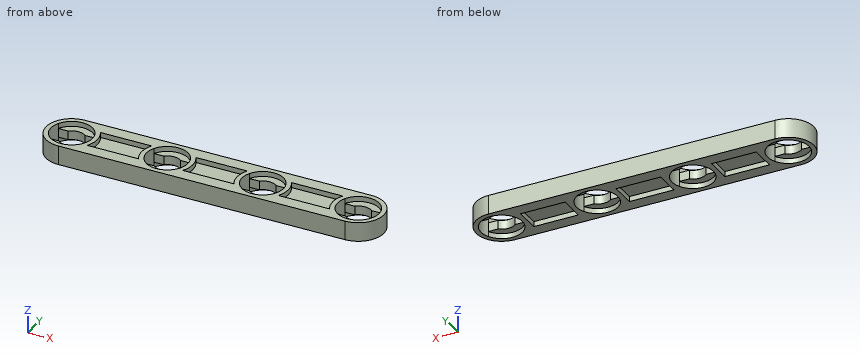
```python
from build123d import *

# Parameters (mm, degrees)
EXTRUDE_1_DEPTH          = 3
CUT_EXTRUDE_1_REACH      = 51.254
SKETCH_3_R               = 3.25
CUT_EXTRUDE_2_DEPTH      = 0.8
CUT_EXTRUDE_START        = -2.2
SKETCH_3_2_R             = 3.25
CUT_EXTRUDE_3_DEPTH      = 0.8
CUT_EXTRUDE_4_DEPTH      = 0.8
SKETCH_5_W               = 7
SKETCH_5_H               = 4
CUT_EXTRUDE_6_DEPTH      = 0.8
MIRROR_2_COPY_1_REACH    = 51.254
MIRROR_2_COPY_2_SKETCH_R = 3.25
MIRROR_2_COPY_2_DEPTH    = 0.8
MIRROR_START             = -2.2
MIRROR_2_COPY_3_SKETCH_R = 3.25
MIRROR_2_COPY_3_DEPTH    = 0.8


with BuildPart() as part:
    # 草图1 → 凸台-拉伸1 (new body)
    with BuildSketch(Plane.XY):
        with BuildLine():
            Line((0, 4), (45, 4))
            ThreePointArc((45, 4), (49, 0), (45, -4))
            Line((45, -4), (0, -4))
            ThreePointArc((0, -4), (-4, 0), (0, 4))
        make_face()
    extrude(amount=-EXTRUDE_1_DEPTH)

    # 草图2 → 切除-拉伸1 (cut, up to next)
    with BuildSketch(Plane.XY, mode=Mode.PRIVATE) as cut_extrude_1_sk1:
        with BuildLine():
            Line((1.322875656, -1.5), (2.883140649, -1.5))
            ThreePointArc((2.883140649, -1.5), (3.25, 0), (2.883140649, 1.5))
            Line((2.883140649, 1.5), (1.322875656, 1.5))
            ThreePointArc((1.322875656, 1.5), (0, 2), (-1.322875656, 1.5))
            Line((-1.322875656, 1.5), (-2.883140649, 1.5))
            ThreePointArc((-2.883140649, 1.5), (-3.25, 0), (-2.883140649, -1.5))
            Line((-2.883140649, -1.5), (-1.322875656, -1.5))
            ThreePointArc((-1.322875656, -1.5), (0, -2), (1.322875656, -1.5))
        make_face()
    cut_extrude_1_tool1 = extrude(cut_extrude_1_sk1.sketch, amount=-CUT_EXTRUDE_1_REACH, mode=Mode.PRIVATE) & part.part
    cut_extrude_1 = cut_extrude_1_tool1.solids().sort_by_distance((0, 0, 0))[0]
    add(cut_extrude_1, mode=Mode.SUBTRACT)

    # 草图3 → 切除-拉伸2 (cut)
    with BuildSketch(Plane.XY):
        Circle(SKETCH_3_R)
    cut_extrude_2 = extrude(amount=-CUT_EXTRUDE_2_DEPTH, mode=Mode.SUBTRACT)

    # 草图3<2> → 切除-拉伸3 (cut)
    with BuildSketch(Plane.XY.offset(CUT_EXTRUDE_START)):
        Circle(SKETCH_3_2_R)
    cut_extrude_3 = extrude(amount=-CUT_EXTRUDE_3_DEPTH, mode=Mode.SUBTRACT)

    # 草图4 → 切除-拉伸4 (cut)
    with BuildSketch(Plane.XY):
        with BuildLine():
            Line((3.464101615, 2), (11.535898385, 2))
            ThreePointArc((11.535898385, 2), (11, 0), (11.535898385, -2))
            Line((11.535898385, -2), (3.464101615, -2))
            ThreePointArc((3.464101615, -2), (4, 0), (3.464101615, 2))
        make_face()
    cut_extrude_4 = extrude(amount=-CUT_EXTRUDE_4_DEPTH, mode=Mode.SUBTRACT)

    # 草图5 → 切除-拉伸6 (cut)
    with BuildSketch(Plane(origin=(0, 0, -3), x_dir=(-1, 0, 0), z_dir=(0, 0, -1))):
        with Locations((-7.5, 0)):
            Rectangle(SKETCH_5_W, SKETCH_5_H)
    cut_extrude_6 = extrude(amount=-CUT_EXTRUDE_6_DEPTH, mode=Mode.SUBTRACT)

    # 镜向1: 切除-拉伸1, 切除-拉伸2, 切除-拉伸3 across plane
    add(cut_extrude_1.mirror(Plane(origin=(7.5, 0, 0), x_dir=(0, 0, 1), z_dir=(1, 0, 0))), mode=Mode.SUBTRACT)
    add(cut_extrude_2.mirror(Plane(origin=(7.5, 0, 0), x_dir=(0, 0, 1), z_dir=(1, 0, 0))), mode=Mode.SUBTRACT)
    add(cut_extrude_3.mirror(Plane(origin=(7.5, 0, 0), x_dir=(0, 0, 1), z_dir=(1, 0, 0))), mode=Mode.SUBTRACT)

    # 镜向2: 切除-拉伸1, 切除-拉伸2, 切除-拉伸3 across plane
    add(cut_extrude_1.mirror(Plane(origin=(22.5, 0, 0), x_dir=(0, 0, 1), z_dir=(1, 0, 0))), mode=Mode.SUBTRACT)
    add(cut_extrude_2.mirror(Plane(origin=(22.5, 0, 0), x_dir=(0, 0, 1), z_dir=(1, 0, 0))), mode=Mode.SUBTRACT)
    add(cut_extrude_3.mirror(Plane(origin=(22.5, 0, 0), x_dir=(0, 0, 1), z_dir=(1, 0, 0))), mode=Mode.SUBTRACT)

    # 镜向2 copy 1 sketch → 镜向2 copy 1 (cut, up to next)
    with BuildSketch(Plane(origin=(30, 0, 0), x_dir=(1, 0, 0), z_dir=(0, 0, 1)), mode=Mode.PRIVATE) as mirror_2_copy_1_sk1:
        with BuildLine():
            Line((1.322875656, -1.5), (2.883140649, -1.5))
            ThreePointArc((2.883140649, -1.5), (3.25, 0), (2.883140649, 1.5))
            Line((2.883140649, 1.5), (1.322875656, 1.5))
            ThreePointArc((1.322875656, 1.5), (0, 2), (-1.322875656, 1.5))
            Line((-1.322875656, 1.5), (-2.883140649, 1.5))
            ThreePointArc((-2.883140649, 1.5), (-3.25, 0), (-2.883140649, -1.5))
            Line((-2.883140649, -1.5), (-1.322875656, -1.5))
            ThreePointArc((-1.322875656, -1.5), (0, -2), (1.322875656, -1.5))
        make_face()
    mirror_2_copy_1_tool1 = extrude(mirror_2_copy_1_sk1.sketch, amount=-MIRROR_2_COPY_1_REACH, mode=Mode.PRIVATE) & part.part
    add(mirror_2_copy_1_tool1.solids().sort_by_distance((30, 0, 0))[0], mode=Mode.SUBTRACT)

    # 镜向2 copy 2 sketch → 镜向2 copy 2 (cut)
    with BuildSketch(Plane(origin=(30, 0, 0), x_dir=(1, 0, 0), z_dir=(0, 0, 1))):
        Circle(MIRROR_2_COPY_2_SKETCH_R)
    extrude(amount=-MIRROR_2_COPY_2_DEPTH, mode=Mode.SUBTRACT)

    # 镜向2 copy 3 sketch → 镜向2 copy 3 (cut)
    with BuildSketch(Plane(origin=(30, 0, 0), x_dir=(1, 0, 0), z_dir=(0, 0, 1)).offset(MIRROR_START)):
        Circle(MIRROR_2_COPY_3_SKETCH_R)
    extrude(amount=-MIRROR_2_COPY_3_DEPTH, mode=Mode.SUBTRACT)

    # 镜向3: 切除-拉伸4, 切除-拉伸6 across plane
    add(cut_extrude_4.mirror(Plane(origin=(15, 0, 0), x_dir=(0, 0, 1), z_dir=(1, 0, 0))), mode=Mode.SUBTRACT)
    add(cut_extrude_6.mirror(Plane(origin=(15, 0, 0), x_dir=(0, 0, 1), z_dir=(1, 0, 0))), mode=Mode.SUBTRACT)

    # 镜向4: 切除-拉伸4, 切除-拉伸6 across plane
    add(cut_extrude_4.mirror(Plane(origin=(22.5, 0, 0), x_dir=(0, 0, 1), z_dir=(1, 0, 0))), mode=Mode.SUBTRACT)
    add(cut_extrude_6.mirror(Plane(origin=(22.5, 0, 0), x_dir=(0, 0, 1), z_dir=(1, 0, 0))), mode=Mode.SUBTRACT)


solid = part.part
```
Build history of the part. All positions in model axes, mm. Coordinates: 2 decimals unless noted, no trailing zeros. Order: outer loops, then holes, each group sorted by start corner. A loop starts at its lowest first (then second) coordinate and runs counter-clockwise, first axis right, second up. Notation, with made-up numbers: M 21.25,-27 L 51.25,-27 A28 cw 51.25,-3 Z; hole C 67.25,-4.75 d2. An arc over 180 degrees is marked long. One line per question, with ' | ' between items. Start each with the question number.
1. Cut at B-B (y = 0). Count the separate pieces of the cut face and the enclosed holes in it, plus the area to 3 significant figures.
2. Cut at A-A (x = 36). Write the cut outline in (y, z), plus the area to 3 significant figures.
3. Wall check: line 1 along Y through (x, z) = (25, -0.05); line 2 along X through (y, z) = (2.5, -2.6); line 3 along X through (y, z) = (-1, -1.95). Give the ranges that are in metal, low to high. Write a range as [from, to].
4. Flat gauge pins, fed straight in: P1, Ø0.5, axis at x = 1, y = 3, coming from the +Z side; P2, Ø0.9, axis at x = 15, y = 2.5, coming from the -Z side; P3, Ø0.9, axis at x = 31, y = 2.5, coming from the +Z side. Where does each tip first touch, or does it go through?
The answers:
1) separate pieces: 5 | enclosed holes: 0 | area: 47.4 mm2
2) outline: M -4,-3 L -2,-3 L -2,-2.2 L 2,-2.2 L 2,-3 L 4,-3 L 4,0 L 2,0 L 2,-0.8 L -2,-0.8 L -2,0 L -4,0 Z | area: 17.6 mm2
3) line 1: y = [-4, -2], [2, 4] | line 2: x = [-3.12, -2.08], [2.08, 12.92], [17.08, 27.92], [32.08, 42.92], [47.08, 48.12] | line 3: x = [-3.87, -3.09], [3.09, 11.91], [18.09, 26.91], [33.09, 41.91], [48.09, 48.87]
4) P1: stops at z = 0 | P2: stops at z = -2.2 | P3: stops at z = -0.8
